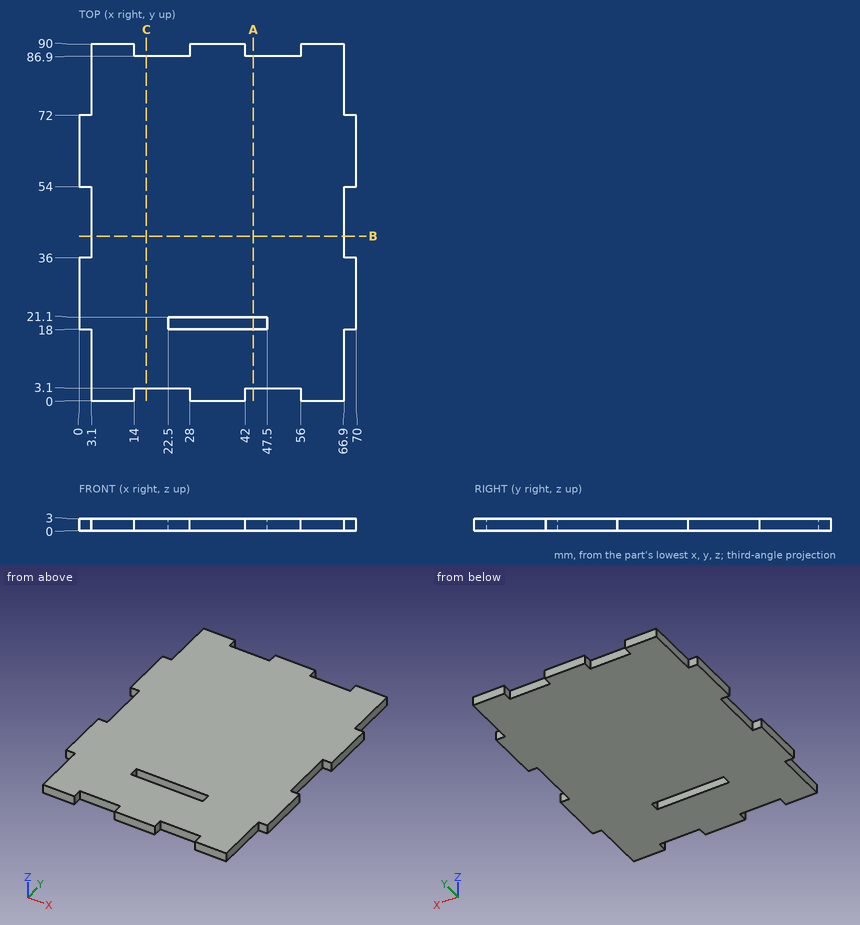
Could you check a few things on this drawing? It's one solid part, dimensions in mm from its lowest x, y, z. Round coordinates to 2 decimals unless told otherwise and drop trailing zeros. Loops run counter-clockwise (first coordinate to the right, second up) from the corner with the lowest first, then second, coordinate; pieces in that order, holes last. Notation, with made-up numbers: (82.25, 30.25) -> (94.25, 30.25) arc R19 ccw to (94.25, 58.25) -> close; hole circle Ø2 at (-4.75, -8). An arc over 180 degrees is marked (long way). Answer as CSV lines item,"result".
1. For pin 1 (0.9 mm diameter, centred on x = 22, z = 1.5, fed in from +Y); pin 2 (1.5 mm diameter, centred on x = 2, z = 2, fed in from -Y); pin 3 (1.5 mm diameter, centred on x = 50, z = 1, fed in from -Y), each with a flat end and sliding along its axis, tell me the tip position at first contact or that it passes through.
Final values:
pin 1,"stops at y = 86.9"
pin 2,"stops at y = 18"
pin 3,"stops at y = 3.1"
2. If we section it at A-A on x = 44: Please give me the cut outline in (y, z), plus the area to 3 significant figures.
Final values:
outline,"(3.1, 0) -> (18, 0) -> (18, 3) -> (3.1, 3) -> close; (21.1, 0) -> (86.9, 0) -> (86.9, 3) -> (21.1, 3) -> close"
area,"242 mm^2"
3. If we section it at B-B on y = 41.5: Please give me the cut outline in (x, z), plus the area to 3 significant figures.
Final values:
outline,"(3.1, 0) -> (66.9, 0) -> (66.9, 3) -> (3.1, 3) -> close"
area,"191 mm^2"
4. If we section it at C-C on x = 17: Please give me the cut outline in (y, z).
Final values:
outline,"(3.1, 0) -> (86.9, 0) -> (86.9, 3) -> (3.1, 3) -> close"
5. If I drill on L1, parallel to Y at x = 23, z = 1; L2, parallel to Y at x = 34, z = 2.75; L3, parallel to X at y = 50.5, z = 1.85, over which ranges is the centre line in solid material (lowest first)?
Final values:
L1,"y = 3.1 to 18, 21.1 to 86.9"
L2,"y = 0 to 18, 21.1 to 90"
L3,"x = 3.1 to 66.9"
